Here's how the part is built. I have some questions about the finished solid (model axes, mm). Face numbers are marked on the shaded views. A direction names the side the tool comes from. Round coordinates to 2 decimals unless told otherwise and drop trailing zeros. Write each loop counter-clockwise with the first axis right and the second up, starting at its lowest first coordinate (ties: lowest second). Pieces come first, ordered by that corner, then holes. Notation, with made-up numbers: (51.5, 1.25) - (56.5, 1.25) arc R16 cw to (56.5, 12.25) - close; hole circle Ø10 at (11, 11.5). An arc over 180 degrees is marked (long way). Write item = value, one per line. Start each with the question number.
Item 1: If we section it at B-B (x = 0.75): Please give me the cut outline in (y, z), and give its area (3 significant figures).
Item 2: If I drill on line 1 along Z through (x, y) = (5, -1); line 2 along Y through (x, z) = (1.75, 1.95); line 3 along Z through (x, y) = (0.25, -2.5), over which ranges is the centre line in solid material (lowest first)? Write a range as [from, to].
Item 3: If we section it at C-C (y = 3): Please give me the cut outline in (x, z).
Item 4: If we section it at D-D (y = -6): Please give me the cut outline in (x, z), and give its area (3 significant figures).
Item 5: If we section it at A-A (z = 0.3): Please give me the cut outline in (x, y).
Item 6: Which directions (+Z, -Z, +X, -X, +Y, -Y) give clear straight access to the entire face, cutting with the end or side of a thin tool? Please do the marked faces 1 and 2.
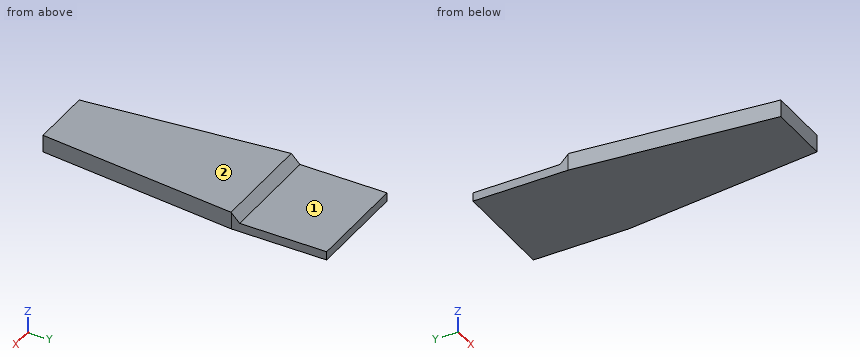
```python
from build123d import *

# Parameters (mm, degrees)
EXTRUDE_1_DEPTH     = 1
EXTRUDE_2_DEPTH     = 6
CUT_EXTRUDE_1_DEPTH = 27.97425922


with BuildPart() as part:
    # 草图1 → 凸台-拉伸1 (new body)
    with BuildSketch(Plane.XY):
        Polygon((6, -3.227529416), (6, 7.720527774), (-6, 7.720527774), (-6, -3.227529416), (-3.598755957, -26.279472226), (3.598755957, -26.279472226), align=None)
    extrude(amount=EXTRUDE_1_DEPTH)

    # 草图2 → 凸台-拉伸2 (add, symmetric)
    with BuildSketch(Plane(origin=(0, 0, 0), x_dir=(0, 0, -1), z_dir=(1, 0, 0))):
        Polygon((-2, -26.279472226), (-1, -26.279472226), (-1, -2.279472226), (-2, -3.279472226), align=None)
    extrude(amount=EXTRUDE_2_DEPTH, both=True)

    # 草图3 → 切除-拉伸1 (cut, through all)
    with BuildSketch(Plane(origin=(0, 0, 1), x_dir=(-1, 0, 0), z_dir=(0, 0, -1))):
        Polygon((6, -26.279472226), (6, -3.227529416), (3.598755957, -26.279472226), align=None)
        Polygon((-6, -26.279472226), (-3.598755957, -26.279472226), (-6, -3.227529416), align=None)
    extrude(amount=-CUT_EXTRUDE_1_DEPTH, mode=Mode.SUBTRACT)


solid = part.part
```
Reply:
q1.outline = (-26.28, 0) - (7.72, 0) - (7.72, 1) - (-2.28, 1) - (-3.28, 2) - (-26.28, 2) - close
q1.area = 57.5 mm2
q2.line_1 = [0, 1]
q2.line_2 = [-26.28, -3.23]
q2.line_3 = [0, 1.22]
q3.outline = (-6, 0) - (6, 0) - (6, 1) - (-6, 1) - close
q4.outline = (-5.71, 0) - (5.71, 0) - (5.71, 2) - (-5.71, 2) - close
q4.area = 22.8 mm2
q5.outline = (-6, -3.23) - (-3.6, -26.28) - (3.6, -26.28) - (6, -3.23) - (6, 7.72) - (-6, 7.72) - close
q6.face_1 = +Z, +X, -X, +Y
q6.face_2 = +Z, +X, -X, +Y, -Y
